Part model, mm, in its own coordinate system. Face numbers are marked on the shaded views. A direction names the side the tool comes from. Round coordinates to 2 decimals unless told otherwise and drop trailing zeros. Write each loop counter-clockwise with the first axis right and the second up, starting at its lowest first coordinate (ties: lowest second). Pieces come first, ordered by that corner, then holes.
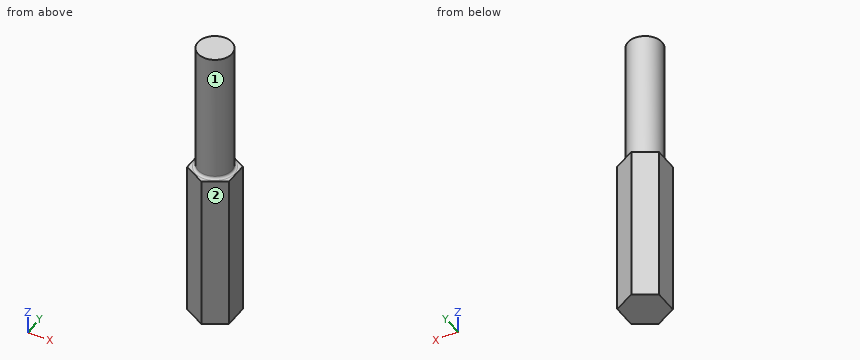
from build123d import *

# Parameters (mm, degrees)
BOSS_EXTRU_1_DEPTH = 30
ESQUISSE2_R        = 3.25
BOSS_EXTRU_2_DEPTH = 25
CONG_1_R           = 0.5


with BuildPart() as part:
    # Esquisse1 → Boss.-Extru.1 (new body)
    with BuildSketch(Plane.XY):
        Polygon((-4, 2.309401077), (-4, -2.309401077), (0, -4.618802154), (4, -2.309401077), (4, 2.309401077), (0, 4.618802154), align=None)
    extrude(amount=BOSS_EXTRU_1_DEPTH)

    # Esquisse2 → Boss.-Extru.2 (add)
    with BuildSketch(Plane.XY.offset(30)):
        Circle(ESQUISSE2_R)
    extrude(amount=BOSS_EXTRU_2_DEPTH)

    # Congé1
    cong_1_edges = [part.edges().sort_by_distance(p)[0] for p in [
        (-3.25, 0, 30),
    ]]
    fillet(cong_1_edges, radius=CONG_1_R)


solid = part.part
Q1. Saw through at A-A, the plane y = 0. Write the cut outline in (x, z), and give its area (3 significant figures).
Q2. Saw through at C-C, the plane z = 43. Write the cut outline in (x, y).
Q3. Tool access for the marked faces 1 and 2: list every direction of +Z, -Z, +X, -X, +Y, -Y with a clear straight run to the whole face (end or side of a thin tool).
Q4. Saw through at B-B, the plane z = 4.5. Write the cut outline in (x, y).
Q5. Wall check: line 1 (Z direction, x = 3.75, y = 1.5); line 2 (X direction, y = 1.75, z = 42.5); line 3 (X direction, y = -3.75, z = 4). Give the ranges that are in metal, low to high.
Q6. Drop flat-ended pins along their axis: P1, Ø1.5, axis at y = 0.5, z = 38, coming from the +X side; P2, Ø5, axis at y = -3.5, z = 47.5, coming from the -X side; P3, Ø1, axis at x = 1, z = 31, coming from the +Y side. Give the stop position or say it passes through.
Computed:
1. outline: (-4, 0) - (4, 0) - (4, 30) - (3.75, 30) arc R0.5 cw to (3.25, 30.5) - (3.25, 55) - (-3.25, 55) - (-3.25, 30.5) arc R0.5 cw to (-3.75, 30) - (-4, 30) - close
1. area: 403 mm2
2. outline: circle Ø6.5 at (0, 0)
3. face 1: +Z
3. face 2: +Z, -Z, +X, -Y
4. outline: (-4, -2.31) - (0, -4.62) - (4, -2.31) - (4, 2.31) - (0, 4.62) - (-4, 2.31) - close
5. line 1: z = 0 to 30
5. line 2: x = -2.74 to 2.74
5. line 3: x = -1.5 to 1.5
6. P1: stops at x = 3.25
6. P2: stops at x = -3.09
6. P3: stops at y = 3.21
